from build123d import *

# Parameters (mm, degrees)
SKETCH1_W           = 20
SKETCH1_H           = 15
BOSS_EXTRUDE1_DEPTH = 4.2
SKETCH2_W           = 8.2
SKETCH2_H           = 10
CUT_EXTRUDE1_DEPTH  = 1
SKETCH3_W           = 8.2
SKETCH3_H           = 8.2
CUT_EXTRUDE2_DEPTH  = 29.564762277
CHAMFER1_SIZE       = 1
SKETCH4_R           = 1.35
CUT_EXTRUDE3_DEPTH  = 29.694000139
CHAMFER2_SIZE       = 5
FILLET1_R           = 4
FILLET2_R           = 1


with BuildPart() as part:
    # Sketch1 → Boss-Extrude1 (new body)
    with BuildSketch(Plane.XY):
        with Locations((10, 12.642136033)):
            Rectangle(SKETCH1_W, SKETCH1_H)
    extrude(amount=BOSS_EXTRUDE1_DEPTH)

    # Sketch2 → Cut-Extrude1 (cut)
    with BuildSketch(Plane.XY.offset(4.2)):
        with Locations((10, 12.642136033)):
            Rectangle(SKETCH2_W, SKETCH2_H)
    extrude(amount=-CUT_EXTRUDE1_DEPTH, mode=Mode.SUBTRACT)

    # Sketch3 → Cut-Extrude2 (cut, through all)
    with BuildSketch(Plane.XY.offset(3.2)):
        with Locations((10, 12.642136033)):
            Rectangle(SKETCH3_W, SKETCH3_H)
    extrude(amount=-CUT_EXTRUDE2_DEPTH, mode=Mode.SUBTRACT)

    # Chamfer1
    chamfer1_edges = [part.edges().sort_by_distance(p)[0] for p in [
        (10, 7.642136033, 4.2),
        (10, 17.642136033, 4.2),
    ]]
    chamfer(chamfer1_edges, length=CHAMFER1_SIZE - 0.0001)  # a hair under: the kernel refuses the full size

    # Sketch4 → Cut-Extrude3 (cut, through all)
    with BuildSketch(Plane.XY.offset(4.2)):
        with Locations((3, 12.642136033)):
            Circle(SKETCH4_R)
        with Locations(Location((17, 12.642136033, 0), (0, 0, 180))):
            Circle(SKETCH4_R)
    extrude(amount=-CUT_EXTRUDE3_DEPTH, mode=Mode.SUBTRACT)

    # Chamfer2
    chamfer2_edges = [part.edges().sort_by_distance(p)[0] for p in [
        (0, 20.142136033, 2.1),
        (20, 20.142136033, 2.1),
        (20, 5.142136033, 2.1),
        (0, 5.142136033, 2.1),
    ]]
    chamfer(chamfer2_edges, length=CHAMFER2_SIZE)

    # Fillet1
    fillet1_edges = [part.edges().sort_by_distance(p)[0] for p in [
        (0, 10.142136033, 2.1),
        (0, 15.142136033, 2.1),
        (15, 20.142136033, 2.1),
        (5, 20.142136033, 2.1),
        (15, 5.142136033, 2.1),
        (5, 5.142136033, 2.1),
        (20, 15.142136033, 2.1),
        (20, 10.142136033, 2.1),
    ]]
    fillet(fillet1_edges, radius=FILLET1_R)

    # Fillet2
    fillet2_edges = [part.edges().sort_by_distance(p)[0] for p in [
        (2.5, 17.642136033, 4.2),
        (10, 20.142136033, 4.2),
        (2.5, 7.642136033, 4.2),
        (10, 5.142136033, 4.2),
        (17.5, 7.642136033, 4.2),
        (20, 12.642136033, 4.2),
        (17.5, 17.642136033, 4.2),
        (0.30448187, 10.268256553, 4.2),
        (5.12612052, 5.446617903, 4.2),
        (14.87387948, 5.446617903, 4.2),
        (19.69551813, 10.268256553, 4.2),
        (19.69551813, 15.016015513, 4.2),
        (14.87387948, 19.837654163, 4.2),
        (5.12612052, 19.837654163, 4.2),
        (0.30448187, 15.016015513, 4.2),
        (0, 12.642136033, 4.2),
    ]]
    fillet(fillet2_edges, radius=FILLET2_R)


solid = part.part
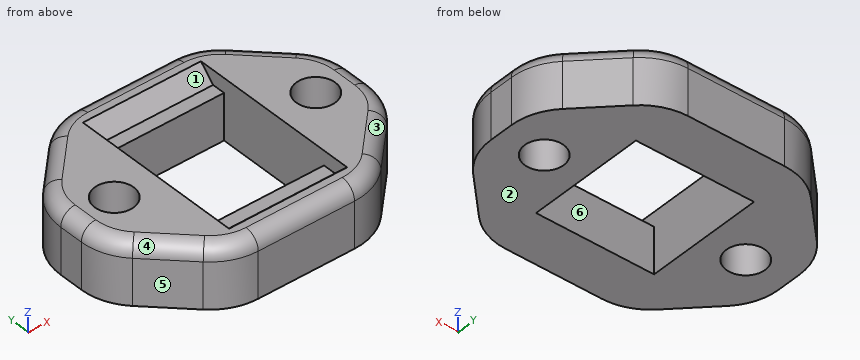
The listing builds one solid part. Answer for the finished solid, in the listing's coordinates (mm). Face numbers are marked on the shaded views. A direction names the side the tool comes from. Give positions to 0.01 mm unless a question says otherwise; leave off trailing zeros. Write each loop counter-clockwise with the first axis right and the second up, starting at its lowest first coordinate (ties: lowest second). Pieces come first, ordered by that corner, then holes.
1) A tool of negligible diameter and unlimited length cuts with its end or side. For the marked faces 5 and 6, from which of +Z, -Z, +X, -X, +Y, -Y can it reach the whole face along a straight path? Write none if from no direction.
2) Find the intervals of material crossed by L1, parallel to Y at x = 13.5, z = 2.35; L2, parallel to X at y = 16.25, z = 2.8; L3, parallel to X at y = 11.25, z = 0.55, in increasing order.
3) Section A-A (y = 12.25) is taken. Write down the section's boundary in (x, z), and give its area (3 significant figures).
4) Given P1, Ø1.3, axis at y = 14, z = 3, coming from the +X side; P2, Ø1, axis at x = 11.5, y = 17.5, coming from the +Z side; P3, Ø1.6, axis at x = 17, y = 12.64, coming from the +Z side; P4, Ø1, axis at y = 14.5, z = 2.5, coming from the -X side, each flat-ended and moving along its own axis, determine where each tip first touches the part or whether it passes through.
5) For a pull along X with two mould halves and no side action, classify the marked faces 1, 2, 3 and 4 as pulls with the +X half, pulls with the -X half, needs draft (parallel to the pull), parting line crosses it, or undercut.
6) Section B-B (z = 2.85) is taken. Write down the section's boundary in (x, y).
Response:
1. face 5: +Z, -Z, -X, -Y
1. face 6: +Z, -Z
2. L1: y = 5.15 to 8.54, 16.74 to 20.14
2. L2: x = 1.11 to 5.9, 14.1 to 18.89
2. L3: x = 0.04 to 5.9, 14.1 to 19.96
3. outline: (0, 0) - (1.71, 0) - (1.71, 4.2) - (1, 4.2) arc R1 ccw to (0, 3.2) - close; (4.29, 0) - (5.9, 0) - (5.9, 4.2) - (4.29, 4.2) - close; (14.1, 0) - (15.71, 0) - (15.71, 4.2) - (14.1, 4.2) - close; (18.29, 0) - (20, 0) - (20, 3.2) arc R1 ccw to (19, 4.2) - (18.29, 4.2) - close
3. area: 27.4 mm2
4. P1: stops at x = 20
4. P2: stops at z = 3.56
4. P3: passes through
4. P4: stops at x = 0.03
5. face 1: undercut
5. face 2: needs draft
5. face 3: pulls with the +X half
5. face 4: pulls with the -X half
6. outline: (0, 11.8) arc R4 ccw to (1.17, 8.97) - (3.83, 6.31) arc R4 ccw to (6.66, 5.14) - (13.34, 5.14) arc R4 ccw to (16.17, 6.31) - (18.83, 8.97) arc R4 ccw to (20, 11.8) - (20, 13.49) arc R4 ccw to (18.83, 16.31) - (16.17, 18.97) arc R4 ccw to (13.34, 20.14) - (6.66, 20.14) arc R4 ccw to (3.83, 18.97) - (1.17, 16.31) arc R4 ccw to (0, 13.49) - close; hole circle Ø2.7 at (3, 12.64); hole (5.9, 8.54) - (14.1, 8.54) - (14.1, 16.74) - (5.9, 16.74) - close; hole circle Ø2.7 at (17, 12.64)
